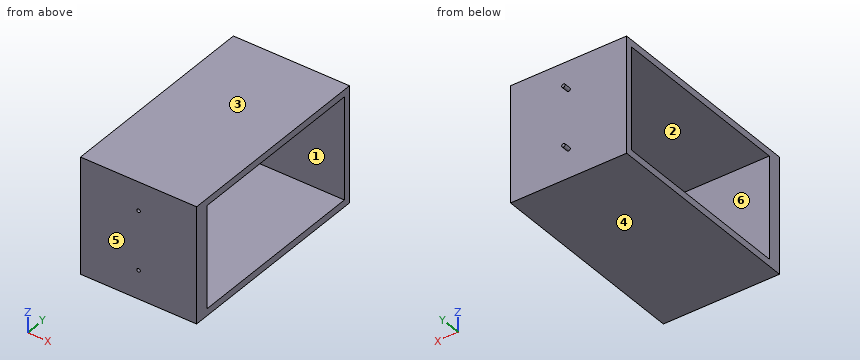
from build123d import *

# Parameters (mm, degrees)
SKETCH1_W           = 50
SKETCH1_H           = 50
BOSS_EXTRUDE2_DEPTH = 89.5
SKETCH4_W           = 44
SKETCH4_H           = 80.5
CUT_EXTRUDE1_DEPTH  = 89.5
SKETCH5_R           = 0.75
CUT_EXTRUDE2_DEPTH  = 3
SKETCH6_R           = 0.75
BOSS_EXTRUDE4_DEPTH = 3


with BuildPart() as part:
    # Sketch1 → Boss-Extrude2 (new body)
    with BuildSketch(Plane(origin=(0, 0, 0), x_dir=(1, 0, 0), z_dir=(0, 1, 0))):
        with Locations((-3.165306342, -9.606735536)):
            Rectangle(SKETCH1_W, SKETCH1_H)
    extrude(amount=BOSS_EXTRUDE2_DEPTH)

    # Sketch4 → Cut-Extrude1 (cut)
    with BuildSketch(Plane(origin=(21.834693658, 0, 0), x_dir=(0, 0, -1), z_dir=(1, 0, 0))):
        with Locations((-9.606735536, 46.25)):
            Rectangle(SKETCH4_W, SKETCH4_H)
    extrude(amount=-CUT_EXTRUDE1_DEPTH, mode=Mode.SUBTRACT)

    # Sketch5 → Cut-Extrude2 (cut)
    with BuildSketch(Plane(origin=(0, 0, 0), x_dir=(-1, 0, 0), z_dir=(0, -1, 0))):
        with Locations(Location((3.165306342, -22.306735536, 0), (0, 0, 90))):
            Circle(SKETCH5_R)
        with Locations(Location((3.165306342, 3.093264464, 0), (0, 0, 90))):
            Circle(SKETCH5_R)
    extrude(amount=-CUT_EXTRUDE2_DEPTH, mode=Mode.SUBTRACT)

    # Sketch6 → Boss-Extrude4 (add)
    with BuildSketch(Plane(origin=(0, 89.5, 0), x_dir=(1, 0, 0), z_dir=(0, 1, 0))):
        with Locations(Location((-3.165306342, 3.093264464, 0), (0, 0, 90))):
            Circle(SKETCH6_R)
        with Locations(Location((-3.165306342, -22.306735536, 0), (0, 0, 90))):
            Circle(SKETCH6_R)
    extrude(amount=BOSS_EXTRUDE4_DEPTH)


solid = part.part
Design review of the part built by this model. Coordinates are the model's own, in mm. Face numbers are marked on the shaded views. A direction names the side the tool comes from. Coordinates: 2 decimals unless noted, no trailing zeros. Write each loop counter-clockwise with the first axis right and the second up, starting at its lowest first coordinate (ties: lowest second). Pieces come first, ordered by that corner, then holes. Notation, with made-up numbers: (39.25, -4) -> (61.25, -4) arc R13 cw to (61.25, 9) -> close; hole circle Ø9 at (-9, 80). An arc over 180 degrees is marked (long way). Write each question's results on one line, items separated by ' | '. Start each with the question number.
(1) Take a section at A-A on z = -5. Write out the cut boundary in (x, y), and give its area (3 significant figures).
(2) Take a section at C-C on x = 14.5. Write out the cut boundary in (y, z).
(3) Take a section at B-B on y = 38. Write out the cut boundary in (x, z), and give its area (3 significant figures).
(4) Tool access review of the marked faces 5 and 6: name each direction out of +Z, -Z, +X, -X, +Y, -Y from which nothing blocks a thin tool from reaching the whole face with its end or side.
(5) For line 1 along Z through (x, y) = (-3, 62); line 2 along Y through (x, z) = (8, -9.5); line 3 along Y through (x, z) = (6, 32.5), list the stretches that pass through material, from the lowest coordinate up. Write a range as from..to.
(6) The part is to be moulded in two halves that separate along Z. For the marked faces 1, 2, 3 and 4, say which applies: pulls with the +Z half, pulls with the -Z half, needs draft (parallel to the pull), parting line crosses it, or undercut.
(7) Clearance check with flat-ended pins moving along their axes: P1, Ø22, axis at x = -6.5, z = 0.5, coming from the -Y side; P2, Ø5, axis at x = -11, z = 19.5, coming from the +Y side; P3, Ø6, axis at y = 81, z = 5, coming from the -X side. State where each tip first meets the part, or that it passes through.
Results found:
1) outline: (-28.17, 0) -> (21.83, 0) -> (21.83, 6) -> (-28.17, 6) -> close; (-28.17, 86.5) -> (21.83, 86.5) -> (21.83, 89.5) -> (-28.17, 89.5) -> close | area: 450 mm2
2) outline: (0, -15.39) -> (89.5, -15.39) -> (89.5, 34.61) -> (0, 34.61) -> close; hole (6, -12.39) -> (86.5, -12.39) -> (86.5, 31.61) -> (6, 31.61) -> close
3) outline: (-28.17, -15.39) -> (21.83, -15.39) -> (21.83, -12.39) -> (-28.17, -12.39) -> close; (-28.17, 31.61) -> (21.83, 31.61) -> (21.83, 34.61) -> (-28.17, 34.61) -> close | area: 300 mm2
4) face 5: +Z, -Z, +X, -X, -Y | face 6: +X, -X
5) line 1: z = -15.39..-12.39, 31.61..34.61 | line 2: y = 0..6, 86.5..89.5 | line 3: y = 0..89.5
6) face 1: undercut | face 2: undercut | face 3: pulls with the +Z half | face 4: pulls with the -Z half
7) P1: stops at y = 0 | P2: stops at y = 89.5 | P3: passes through
